For this review, take the finished solid that the model builds, in its own axes (mm). Round coordinates to 2 decimals unless told otherwise and drop trailing zeros. Write each loop counter-clockwise with the first axis right and the second up, starting at its lowest first coordinate (ties: lowest second). Pieces come first, ordered by that corner, then holes.
from build123d import *

# Parameters (mm, degrees)
F0_W     = 80
F0_H     = 80
F1_DEPTH = 80
F3_R     = 5
F2_R     = 10.8374332622
F4_DEPTH = 80.001


with BuildPart() as f1:
    # F0 (on Top) → F1 (new body)
    with BuildSketch(Plane.XY):
        with Locations((-41.452800855, 28.8035999984)):
            Rectangle(F0_W, F0_H)
    extrude(amount=F1_DEPTH)

    # F3
    f3_edges = [f1.edges().sort_by_distance(p)[0] for p in [
        (-81.452801, -11.1964, 40),
        (-1.452801, -11.1964, 40),
        (-1.452801, 68.8036, 40),
        (-81.452801, 68.8036, 40),
        (-81.452801, 28.8036, 0),
        (-81.452801, 28.8036, 80),
    ]]
    fillet(f3_edges, radius=F3_R)

    # F2 (on face) → F4 (cut, through all)
    with BuildSketch(Plane.XY.offset(80)):
        with Locations((-41.9264025986, 33.4499999881)):
            Circle(F2_R)
    extrude(amount=-F4_DEPTH, mode=Mode.SUBTRACT)


solid = f1.part
(1) We need section C-C, the plane y = 42.5. Give the boundary of the cut face in (x, z), and give its area (3 significant figures).
Geometry check:
outline: (-81.45, 5) arc R5 ccw to (-76.45, 0) - (-47.89, 0) - (-47.89, 80) - (-76.45, 80) arc R5 ccw to (-81.45, 75) - close; (-35.96, 0) - (-1.45, 0) - (-1.45, 80) - (-35.96, 80) - close
area: 5,440 mm2
(2) For pin 1 Ø1.5 at (x, y) = (-46.5, 25.5) entering from +Z, flat-tipped, find the tip position at first contact; note if it passes through.
Geometry check:
pin 1: passes through
(3) We need section B-B, the plane z = 58. Give the boundary of the cut face in (x, y), and give its area (3 significant figures).
Geometry check:
outline: (-81.45, -6.2) arc R5 ccw to (-76.45, -11.2) - (-6.45, -11.2) arc R5 ccw to (-1.45, -6.2) - (-1.45, 63.8) arc R5 ccw to (-6.45, 68.8) - (-76.45, 68.8) arc R5 ccw to (-81.45, 63.8) - close; hole circle Ø21.67 at (-41.93, 33.45)
area: 6,010 mm2
(4) Mouldability with a two-part tool opening along X and no side actions: class faces 1 (the face through (-36.926, 23.835, 40.56)), 2 (the face through (-42, -11.196, 39)), 3 (the face through (-2.88, 67.3, 40.56)), 4 (the face through (-80.027, 67.3, 40.56)) as pulls with the +X half, pulls with the -X half, needs draft (parallel to the pull), parting line crosses it, or undercut.
Geometry check:
face 1: undercut
face 2: needs draft
face 3: pulls with the +X half
face 4: pulls with the -X half
(5) For line 1 along X through (y, z) = (33, 43); line 2 along X through (y, z) = (25, 37); line 3 along Y through (x, z) = (-47, 49), list the stretches that pass through material, from the lowest coordinate up.
Geometry check:
line 1: x = -81.45 to -52.75, -31.1 to -1.45
line 2: x = -81.45 to -48.71, -35.14 to -1.45
line 3: y = -11.2 to 23.87, 43.03 to 68.8
(6) We need section A-A, the plane y = 33.45. Give the boundary of the cut face in (x, z).
Geometry check:
outline: (-81.45, 5) arc R5 ccw to (-76.45, 0) - (-52.76, 0) - (-52.76, 80) - (-76.45, 80) arc R5 ccw to (-81.45, 75) - close; (-31.09, 0) - (-1.45, 0) - (-1.45, 80) - (-31.09, 80) - close
